```python
from build123d import *

# Parameters (mm, degrees)
SKETCH_W        = 29
SKETCH_H        = 47
PAD_DEPTH       = 40
SKETCH001_R     = 9.75
PAD001_DEPTH    = 10
SKETCH002_W     = 56
SKETCH002_H     = 6
POCKET_DEPTH    = 100
SKETCH003_W     = 54.44
SKETCH003_H     = 5.76
POCKET001_DEPTH = 40.001
SKETCH004_R     = 1.1
POCKET002_DEPTH = 5
SKETCH005_R     = 3.5
POCKET003_DEPTH = 2
SKETCH006_W     = 40
SKETCH006_H     = 20
PAD002_DEPTH    = 10
FILLET_R        = 9
FILLET001_R     = 9
SKETCH007_R     = 2.5
POCKET004_DEPTH = 40.001


with BuildPart() as part:
    # Sketch → Pad (new body)
    with BuildSketch(Plane.XY.offset(10)):
        with BuildLine():
            Line((0, 0), (40, 0))
            Line((40, 0), (40, 60))
            ThreePointArc((40, 60), (20, 68.990653), (0, 60))
            Line((0, 60), (0, 0))
        make_face()
        with Locations((20, 30)):
            Rectangle(SKETCH_W, SKETCH_H, mode=Mode.SUBTRACT)
    extrude(amount=PAD_DEPTH)

    # Sketch001 (on Face9 of Pad) → Pad001 (join)
    with BuildSketch(Plane(origin=(0, 0, 10), x_dir=(1, 0, 0), z_dir=(0, 0, -1))):
        with BuildLine():
            Line((40, -60), (40, 30))
            ThreePointArc((40, 30), (20, 50), (0, 30))
            Line((0, 30), (0, -60))
            ThreePointArc((0, -60), (20, -68.990653), (40, -60))
        make_face()
        with Locations((20, -42.25)):
            Circle(SKETCH001_R, mode=Mode.SUBTRACT)
    extrude(amount=PAD001_DEPTH)

    # Sketch002 (on Face7 of Pad001) → Pocket (cut)
    with BuildSketch(Plane(origin=(0, 0, 0), x_dir=(0, -1, 0), z_dir=(-1, 0, 0))):
        with Locations((-48, 3)):
            Rectangle(SKETCH002_W, SKETCH002_H)
    extrude(amount=-POCKET_DEPTH, mode=Mode.SUBTRACT)

    # Sketch003 (on Face8 of Pocket) → Pocket001 (cut, through all)
    with BuildSketch(Plane.YZ.offset(40)):
        with Locations((-27.22, 7.88)):
            Rectangle(SKETCH003_W, SKETCH003_H)
    extrude(amount=-POCKET001_DEPTH, mode=Mode.SUBTRACT)

    # Sketch004 (on Face12 of Pocket001) → Pocket002 (cut)
    with BuildSketch(Plane(origin=(0, 0, 0), x_dir=(1, 0, 0), z_dir=(0, 0, -1))):
        with Locations((11.98, 30)):
            Circle(SKETCH004_R)
        with Locations((14.34, 35.7)):
            Circle(SKETCH004_R)
        with Locations((20, 37.98)):
            Circle(SKETCH004_R)
        with Locations((25.66, 35.7)):
            Circle(SKETCH004_R)
        with Locations((28.02, 30)):
            Circle(SKETCH004_R)
        with Locations((25.66, 24.34)):
            Circle(SKETCH004_R)
        with Locations((20, 22.02)):
            Circle(SKETCH004_R)
        with Locations((14.34, 24.34)):
            Circle(SKETCH004_R)
    extrude(amount=-POCKET002_DEPTH, mode=Mode.SUBTRACT)

    # Sketch005 (on Face7 of Pocket002) → Pocket003 (cut)
    with BuildSketch(Plane.XY.offset(5)):
        with Locations((20, -30)):
            Circle(SKETCH005_R)
    extrude(amount=-POCKET003_DEPTH, mode=Mode.SUBTRACT)

    # Sketch006 (on Face12 of Pocket003) → Pad002 (join)
    with BuildSketch(Plane(origin=(0, 0, 0), x_dir=(1, 0, 0), z_dir=(0, 0, -1))):
        with Locations((20, -10)):
            Rectangle(SKETCH006_W, SKETCH006_H)
    extrude(amount=PAD002_DEPTH)

    # Fillet
    fillet_edges = [part.edges().sort_by_distance(p)[0] for p in [
        (20, 20, -10),
    ]]
    fillet(fillet_edges, radius=FILLET_R)

    # Fillet001
    fillet001_edges = [part.edges().sort_by_distance(p)[0] for p in [
        (20, 0, -10),
    ]]
    fillet(fillet001_edges, radius=FILLET001_R)

    # Sketch007 (on Face8 of Fillet001) → Pocket004 (cut, through all)
    with BuildSketch(Plane(origin=(0, 0, 0), x_dir=(0, -1, 0), z_dir=(-1, 0, 0))):
        with Locations((-10, -5)):
            Circle(SKETCH007_R)
    extrude(amount=-POCKET004_DEPTH, mode=Mode.SUBTRACT)


solid = part.part
```
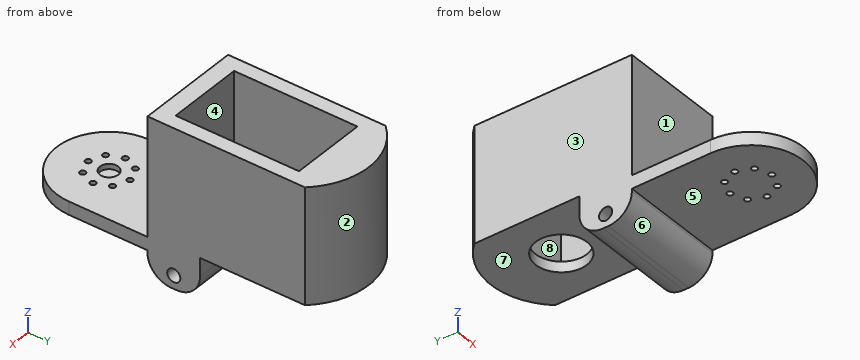
The model under review builds one solid part; all positions refer to its coordinate system, in mm. Face numbers are marked on the shaded views. A direction names the side the tool comes from. Coordinates: 2 decimals unless noted, no trailing zeros. Order: outer loops, then holes, each group sorted by start corner. A loop starts at its lowest first (then second) coordinate and runs counter-clockwise, first axis right, second up. Notation, with made-up numbers: M 18,0.5 L 63,0.5 A20 ccw 63,32.5 Z; hole C 48.5,-7.5 d3. An arc over 180 degrees is marked long. One line per question, with ' | ' between items.
(1) Insertion check: pin 1 (1.5 mm diameter, centred on x = 27.5, z = -3.5, fed in from +Y); pin 2 (12 mm diameter, centred on x = 11.5, y = -32.5, fed in from -Z); pin 3 (23 mm diameter, centred on x = 23.5, y = 21, fed in from +Z); pin 4 (7.5 mm diameter, centred on x = 13.5, z = 4, fed in from +Y). Each pin has a flat end and moves straight along its axis. Give the tip position at first contact, or say it passes through.
Geometry results:
pin 1: stops at y = 19.83 | pin 2: stops at z = 0 | pin 3: stops at z = 50 | pin 4: stops at y = 68.78
(2) Add section D-D, the plane y = 14. Write out the cut boundary in (x, z).
Geometry results:
outline: M 0,-9.49 L 40,-9.49 L 40,50 L 34.5,50 L 34.5,10 L 5.5,10 L 5.5,50 L 0,50 Z
(3) The part is to be moulded in two halves that separate along Y. For the marked faces 6, 7 and 8, say which applies: +Y half, -Y half, draft (parallel to the pull), parting line (faces both ways), or undercut.
Geometry results:
face 6: -Y half | face 7: draft | face 8: undercut
(4) Add section A-A, the plane z = -5. Write out the cut boundary in (x, y), then the cut area to 3 significant figures.
Geometry results:
outline: M 0,0.94 L 40,0.94 L 40,7.5 L 0,7.5 Z; M 0,12.5 L 40,12.5 L 40,19.06 L 0,19.06 Z | area: 525 mm²
(5) For probe 1 along X at (y, z) = (28.5, 17); probe 2 along Y at (x, z) = (14, 2); probe 3 along X at (y, z) = (-35, 3), list the stretches that pass through material, from the lowest coordinate up. Write a range as from..to.
Geometry results:
probe 1: x = 0..5.5, 34.5..40 | probe 2: y = -49.08..-36.75, -34.65..-25.39, -23.29..20 | probe 3: x = 0.64..13.49, 15.19..24.81, 26.51..39.36
(6) Machinability: for the marked faces 1, 2, 3, 4 and 5, which of the approach directions +Z, -Z, +X, -X, +Y, -Y give a long, thin tool a straight path to every point of the face, cutting with its end or side? Answer none if there is none.
Geometry results:
face 1: +Z, +X, -X, -Y | face 2: +Z, -Z, +Y | face 3: +Z, -Z, -X, +Y, -Y | face 4: +Z | face 5: -Z, +X, -X, -Y
(7) Add section C-C, the plane x = 37. Write out the cut boundary in (y, z).
Geometry results:
outline: M -40.54,0 L 0,0 L 0,-1 A9 ccw 9,-10 L 11,-10 A9 ccw 20,-1 L 20,6 L 62.89,6 L 62.89,50 L 0,50 L 0,5 L -40.54,5 Z; hole C 10,-5 d5
(8) Add section B-B, the plane y = 50.5. Write out the cut boundary in (x, z).
Geometry results:
outline: M 0,6 L 14.8,6 L 14.8,10 L 5.5,10 L 5.5,50 L 0,50 Z; M 25.2,6 L 40,6 L 40,50 L 34.5,50 L 34.5,10 L 25.2,10 Z
